from build123d import *

# Parameters (mm, degrees)
F0_R     = 11.43
F1_DEPTH = 774.7
F2_R     = 17.78
F3_DEPTH = 25.4
F4_DEPTH = 48.26
F5_R     = 1.2732150617
F6_DEPTH = 2.54
F6_TAPER = 15


with BuildPart() as f1:
    # F0 (on Top) → F1 (new body)
    with BuildSketch(Plane.XY):
        Circle(F0_R)
    extrude(amount=F1_DEPTH)

    # F2 (on face) → F3 (join)
    with BuildSketch(Plane(origin=(0, 0, 0), x_dir=(1, 0, 0), z_dir=(0, 0, -1))):
        Circle(F2_R)
    extrude(amount=F3_DEPTH)

    # F4 (cut): a face of the model
    f4_faces = [f1.faces().sort_by_distance(p)[0] for p in [
        (0, 0, 774.7),
    ]]
    extrude(f4_faces, amount=-F4_DEPTH, mode=Mode.SUBTRACT)

    # F5 (on face) → F6 (cut)
    with BuildSketch(Plane(origin=(0, 0, -25.4), x_dir=(1, 0, 0), z_dir=(0, 0, -1))):
        Circle(F5_R)
    extrude(amount=-F6_DEPTH, taper=F6_TAPER, mode=Mode.SUBTRACT)


solid = f1.part
Here's how the part is built. I have some questions about the finished solid (model axes, mm). A direction names the side the tool comes from. Coordinates: 2 decimals unless noted, no trailing zeros. Order: outer loops, then holes, each group sorted by start corner. A loop starts at its lowest first (then second) coordinate and runs counter-clockwise, first axis right, second up. Notation, with made-up numbers: M 5,-5 L 47,-5 A30 ccw 47,31 Z; hole C -9,-15.75 d7. An arc over 180 degrees is marked long. Answer as CSV lines item,"result".
Item 1: Imagine slicing it at A-A on z = 554.5. Write out the boundary of the cut face in (x, y).
Results found:
outline,"C 0,0 d22.86"
Item 2: If I drill on line 1 (Z direction, x = 13.5, y = 4); line 2 (X direction, y = 1.5, z = 334.5); line 3 (Y direction, x = 1, z = 106), over which ranges is the centre line in solid material (lowest first)?
Results found:
line 1,"-25.4 to 0"
line 2,"-11.33 to 11.33"
line 3,"-11.39 to 11.39"
Item 3: For pin 1 (5 mm diameter, centred on x = 6.5, y = 9.5, fed in from +Z); pin 2 (12 mm diameter, centred on x = -2.5, z = 139, fed in from -Y); pin 3 (6 mm diameter, centred on y = -11, z = 277, fed in from -X); pin 4 (2 mm diameter, centred on x = -12.5, y = 2.5, fed in from +Z), each with a flat end and sliding along its axis, tell me the tip position at first contact or that it passes through.
Results found:
pin 1,"z = 726.44"
pin 2,"y = -11.43"
pin 3,"x = -8.16"
pin 4,"z = 0"
Item 4: On a 3-axis mill with a long thin cutter (end or side, diameter ignored), from which of +Z, -Z, +X, -X, +Y, -Y can I reach the whole of each face in a straight line? I mean faces 1 (the face through (10.902, 3.433, 358.135)), 2 (the face through (0, 4, -25.4)). Say none if no direction works.
Results found:
face 1,"+Z"
face 2,"-Z, +X, -X, +Y, -Y"
